Geometry: final body of the model. Coordinates: model frame, mm. Face numbers are marked on the shaded views. A direction names the side the tool comes from. Give positions to 0.01 mm unless a question says otherwise; leave off trailing zeros. Loops run counter-clockwise (first coordinate to the right, second up) from the corner with the lowest first, then second, coordinate; pieces in that order, holes last. Notation, with made-up numbers: M 87.5,29.25 L 145.5,29.25 A28 cw 145.5,49.25 Z; hole C -20.5,83.25 d7. An arc over 180 degrees is marked long. Put each result on its own line as item: value.
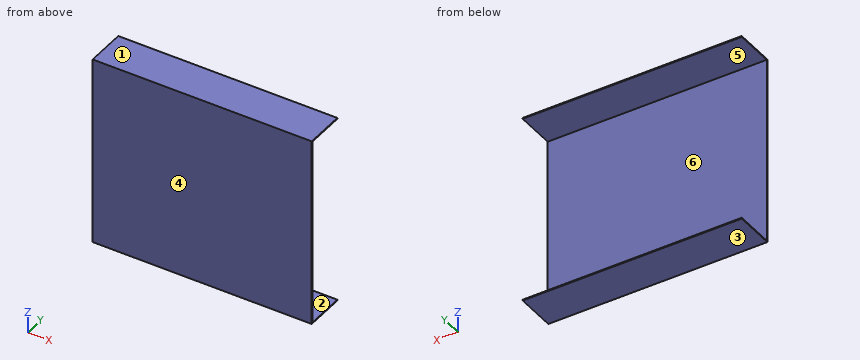
```python
from build123d import *

# Parameters (mm, degrees)
CROQUIS1_W              = 120
CROQUIS1_H              = 25
SALIENTE_EXTRUIR1_DEPTH = 140
VACIADO1_T              = 0.6


with BuildPart() as part:
    # Croquis1 → Saliente-Extruir1 (new body)
    with BuildSketch(Plane(origin=(0, 0, 0), x_dir=(0, 0, -1), z_dir=(1, 0, 0))):
        with Locations((60, 12.5)):
            Rectangle(CROQUIS1_W, CROQUIS1_H)
    extrude(amount=SALIENTE_EXTRUIR1_DEPTH)

    # Vaciado1
    vaciado1_openings = [part.faces().sort_by_distance(p)[0] for p in [
        (70, 25, -60),
        (0, 12.5, -60),
        (140, 12.5, -60),
    ]]
    offset(amount=VACIADO1_T, openings=vaciado1_openings, kind=Kind.INTERSECTION)


solid = part.part
```
Item 1: Line query: probe 1 along Z at (x, y) = (91, 14.75); probe 2 along Y at (x, z) = (18, -15.5). Output: solid intervals per line, ascending. Write a range as [from, to].
Output values:
probe 1: [-120.6, -120], [0, 0.6]
probe 2: [-0.6, 0]
Item 2: Mould query, pull axis Z, two halves, no side actions, for the marked faces 3, 4, 5 and 6. Classes: pulls with the +Z half, pulls with the -Z half, needs draft (parallel to the pull), parting line crosses it, or undercut.
Output values:
face 3: pulls with the -Z half
face 4: needs draft
face 5: undercut
face 6: undercut
Item 3: Set-up query: the marked faces 1 and 2. Return all of +Z, -Z, +X, -X, +Y, -Y with unobstructed straight access to the full face (end or side cutting, diameter ignored); none if empty.
Output values:
face 1: +Z, +X, -X, +Y, -Y
face 2: +X, -X, +Y
Item 4: Section B-B on x = 74. Output: boundary loops of the cut face in (y, z), then the cut area to 3 significant figures.
Output values:
outline: M -0.6,-120.6 L 25,-120.6 L 25,-120 L 0,-120 L 0,0 L 25,0 L 25,0.6 L -0.6,0.6 Z
area: 103 mm²
Item 5: Pin query (flat end, axial travel): pin 1 Ø10 at (x, z) = (118, -88.5) entering from +Y. Return the tip coordinate at first contact, or that it passes through.
Output values:
pin 1: y = 0
Item 6: Section C-C on z = -12.5. Output: boundary loops of the cut face in (x, y), then the cut area to 3 significant figures.
Output values:
outline: M 0,-0.6 L 140,-0.6 L 140,0 L 0,0 Z
area: 84.0 mm²
Item 7: Section A-A on y = 23.25. Output: boundary loops of the cut face in (x, z).
Output values:
outline: M 0,-120.6 L 140,-120.6 L 140,-120 L 0,-120 Z; M 0,0 L 140,0 L 140,0.6 L 0,0.6 Z
